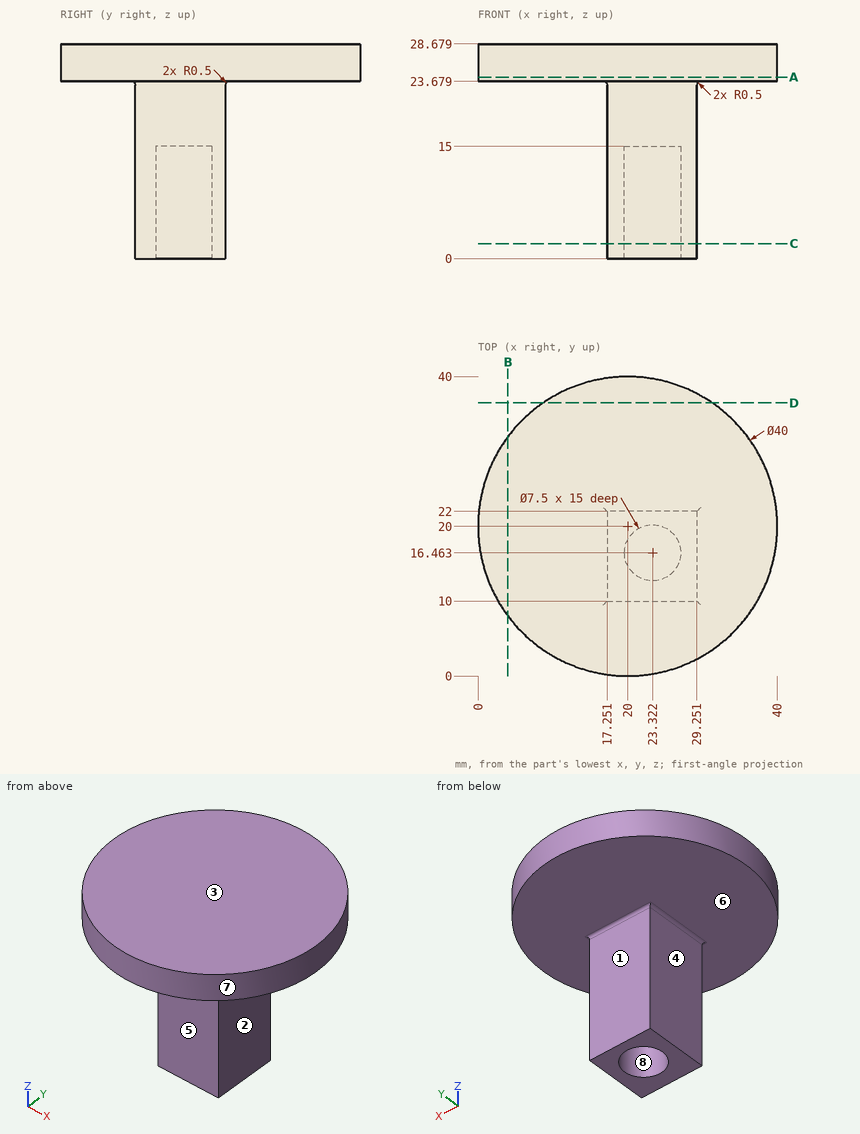
Answer from the drawing. Dimensions are ordinates in mm from the lowest x, y and z of the part. A direction names the side the tool comes from. Coordinates: 2 decimals unless noted, no trailing zeros. Loops run counter-clockwise (first coordinate to the right, second up) from the corner with the lowest first, then second, coordinate; pieces in that order, holes last.
Q1. The mould has two halves that part along Y. Classify the marked faces 6, 7 and 8: +Y half, -Y half, draft (parallel to the pull), parting line (faces both ways), or undercut.
Q2. The part is cut by section C-C on z = 2. Write down the section's boundary in (x, y).
Q3. Consider probe 1 along Z at (x, y) = (18, 37.5); probe 2 along Y at (x, z) = (24.5, 19.5); probe 3 along X at (y, z) = (20.5, 11.75). Determine where each line is inside the solid, lowest interval first.
Q4. The part is cut by section B-B on x = 4. Write down the section's boundary in (y, z), and give its area (3 significant figures).
Q5. The part is cut by section D-D on y = 36.5. Write down the section's boundary in (x, z), and give its area (3 significant figures).
Q6. Which of the six approach directions +Z, -Z, +X, -X, +Y, -Y give full straight-line access (tool end or side, diameter ignored) to the marked faces 1, 2, 3, 4 and 5?
Q7. Each of these flat-tipped pins is pushed along its axis until it touches: pin 1 Ø3.5 at (y, z) = (14.5, 15.5) entering from +X; pin 2 Ø9.5 at (x, z) = (23.5, 7.5) entering from +Y; pin 3 Ø10 at (x, y) = (12, 26.5) entering from -Z. Where does it stop, or does it pass through?
Q8. The part is cut by section A-A on z = 24.25. Write down the section's boundary in (x, y), and give its area (3 significant figures).
Results below:
1. face 6: draft
1. face 7: parting line
1. face 8: undercut
2. outline: (17.25, 10) - (29.25, 10) - (29.25, 22) - (17.25, 22) - close; hole circle Ø7.5 at (23.32, 16.46)
3. probe 1: z = 23.68 to 28.68
3. probe 2: y = 10 to 22
3. probe 3: x = 17.25 to 29.25
4. outline: (8, 23.68) - (32, 23.68) - (32, 28.68) - (8, 28.68) - close
4. area: 120 mm2
5. outline: (8.7, 23.68) - (31.3, 23.68) - (31.3, 28.68) - (8.7, 28.68) - close
5. area: 113 mm2
6. face 1: -Z, +X, -X, +Y
6. face 2: -Z, +X, +Y, -Y
6. face 3: +Z, +X, -X, +Y, -Y
6. face 4: -Z, -X, +Y, -Y
6. face 5: -Z, +X, -X, -Y
7. pin 1: stops at x = 29.25
7. pin 2: stops at y = 22
7. pin 3: stops at z = 23.68
8. outline: circle Ø40 at (20, 20)
8. area: 1,260 mm2
